Job drawing, mm, ordinate dimensions from the low corner. One solid piece. A direction names the side the tool comes from. Round coordinates to 2 decimals unless told otherwise and drop trailing zeros. Loops run counter-clockwise (first coordinate to the right, second up) from the corner with the lowest first, then second, coordinate; pieces in that order, holes last.
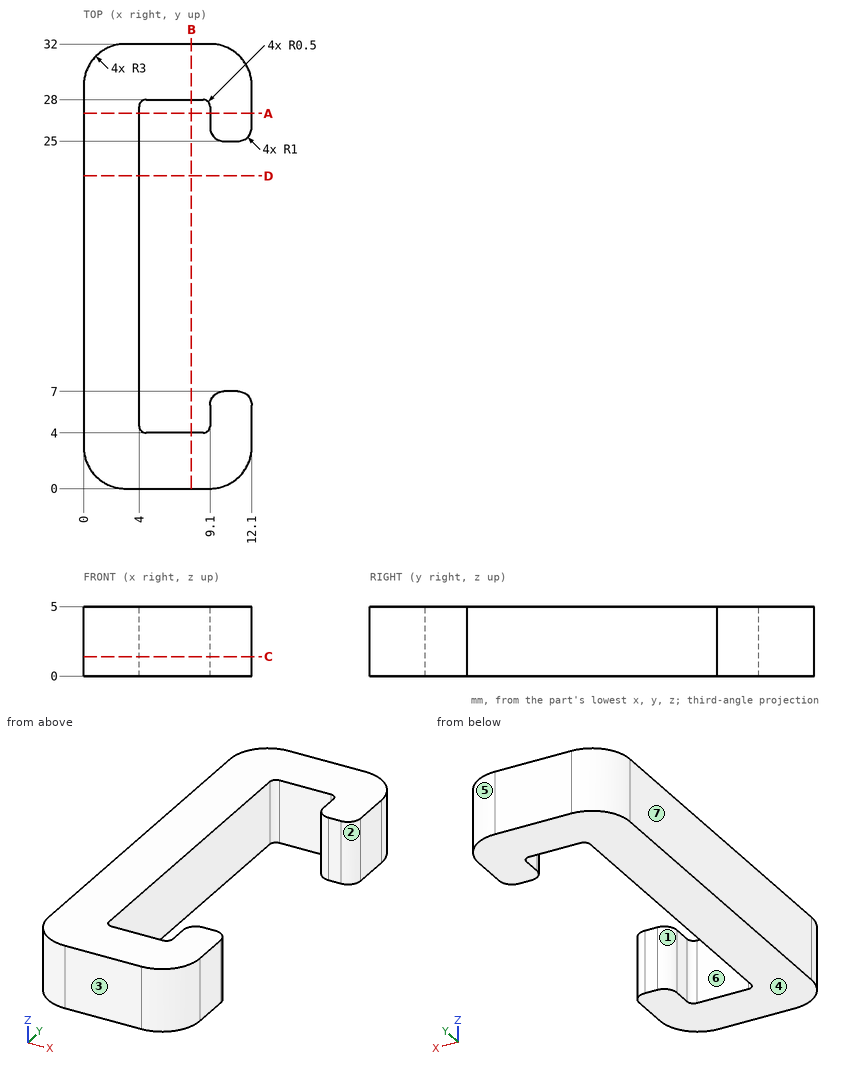
1) Drop flat-ended pins along their axis: pin 1 Ø0.5 at (x, z) = (10.5, 3) entering from -Y; pin 2 Ø3 at (x, y) = (6, 10.5) entering from +Z (3 decimals); pin 3 Ø1.5 at (y, z) = (18, 3.5) entering from +X; pin 4 Ø1.1 at (x, z) = (10.5, 1.5) entering from +Y. Give the stop position or say it passes through.
Values:
pin 1: stops at y = 0.23
pin 2: passes through
pin 3: stops at x = 4
pin 4: stops at y = 31.88
2) Wall check: line 1 along Y through (x, z) = (8.25, 4.4); line 2 along X through (y, z) = (5, 4.85); line 3 along X through (y, z) = (15, 3.3). Give the ranges that are in metal, low to high.
Values:
line 1: y = 0 to 4, 28 to 32
line 2: x = 0 to 4, 9.1 to 12.1
line 3: x = 0 to 4
3) Slice it at C-C, the plane z = 1.4. Give the cut face in (x, y).
Values:
outline: (0, 3) arc R3 ccw to (3, 0) - (9.1, 0) arc R3 ccw to (12.1, 3) - (12.1, 6) arc R1 ccw to (11.1, 7) - (10.1, 7) arc R1 ccw to (9.1, 6) - (9.1, 4.5) arc R0.5 cw to (8.6, 4) - (4.5, 4) arc R0.5 cw to (4, 4.5) - (4, 27.5) arc R0.5 cw to (4.5, 28) - (8.6, 28) arc R0.5 cw to (9.1, 27.5) - (9.1, 26) arc R1 ccw to (10.1, 25) - (11.1, 25) arc R1 ccw to (12.1, 26) - (12.1, 29) arc R3 ccw to (9.1, 32) - (3, 32) arc R3 ccw to (0, 29) - close
4) Tool access for the marked faces 1, 2 and 3: list every direction of +Z, -Z, +X, -X, +Y, -Y with a clear straight run to the whole face (end or side of a thin tool).
Values:
face 1: +Z, -Z
face 2: +Z, -Z, +X
face 3: +Z, -Z, +X, -X, -Y
5) Slice it at B-B, the plane x = 7.75. Give the cut face in (y, z).
Values:
outline: (0, 0) - (4, 0) - (4, 5) - (0, 5) - close; (28, 0) - (32, 0) - (32, 5) - (28, 5) - close
6) Slice it at D-D, the plane y = 22.5. Give the cut face in (x, z), then the cut area to 3 significant figures.
Values:
outline: (0, 0) - (4, 0) - (4, 5) - (0, 5) - close
area: 20.0 mm2
7) Slice it at A-A, the plane y = 27. Give the cut face in (x, z), then the cut area to 3 significant figures.
Values:
outline: (0, 0) - (4, 0) - (4, 5) - (0, 5) - close; (9.1, 0) - (12.1, 0) - (12.1, 5) - (9.1, 5) - close
area: 35.0 mm2
8) Mould opens along X. For the marked faces 4, 5, 6 and 7 say: released by +X, released by -X, zero draft, split by the parting line, or undercut.
Values:
face 4: zero draft
face 5: released by +X
face 6: undercut
face 7: released by -X
